Autodesk Inventor part; units mm, degrees
ref_plane "YZ Plane" through (0, 0, 0) normal (1, 0, 0) x (0, 1, 0)
ref_plane "XZ Plane" through (0, 0, 0) normal (0, 1, 0) x (-1, 0, 0)
ref_plane "XY Plane" through (0, 0, 0) normal (0, 0, 1) x (1, 0, 0)
sketch "Sketch1" plane through (0, 0, 0) normal (0, 1, 0) x (-1, 0, 0)
  line L0 (8.2338, 13.4805) -> (-21.7662, 13.4805)
  line L1 (-21.7662, 13.4805) -> (-21.7662, -11.5195)
  line L2 (-21.7662, -11.5195) -> (8.2338, -11.5195)
  line L3 (8.2338, -11.5195) -> (8.2338, 13.4805)
  point P0 (0, 0)
  dimension "d0" = 25
  dimension "d1" = 30
extrude "Extrusion1" add sketch "Sketch1" along normal blind 12.7
sketch "Sketch2" plane through (0, 0, 0) normal (0, -1, 0) x (1, 0, 0)
  line L0 (-8.2338, 13.4805) -> (21.7662, 13.4805)
  line L1 (21.7662, 13.4805) -> (21.7662, -11.5195)
  point P0 (0, 0)
  point P1 (19.2262, 10.3055)
  point P2 (19.2262, -8.7445)
  point P3 (-6.1738, -8.7445)
  point P4 (-6.1738, 10.3055)
  dimension "d4" = 3.175
  dimension "d5" = 2.54
  dimension "d6" = 19.05
  dimension "d7" = 2.54
  dimension "d8" = 25.4
  dimension "d9" = 3.175
  dimension "d10" = 19.05
  dimension "d11" = 0
hole "Hole1" at (19.2262, 0, 10.3055) at (19.2262, 0, -8.7445) at (-6.1738, 0, -8.7445) at (-6.1738, 0, 10.3055) direction (0, 1, 0) diameter 2.6416 depth 10 tip angle 118.188
sketch "Sketch3" plane through (0, 12.7, 0) normal (0, 1, 0) x (1, 0, 0)
  line L0 (-4.3838, -10.8805) -> (17.9162, -10.8805)
  line L1 (17.9162, -10.8805) -> (17.9162, 8.9195)
  line L2 (17.9162, 8.9195) -> (-4.3838, 8.9195)
  line L3 (-4.3838, 8.9195) -> (-4.3838, -10.8805)
  line L4 (-8.2338, 11.5195) -> (-8.2338, -13.4805)
  line L5 (21.7662, 11.5195) -> (-8.2338, 11.5195)
  point P0 (0, 0)
  dimension "d19" = 19.8
  dimension "d20" = 22.3
  dimension "d22" = 3.85
  dimension "d23" = 2.6
extrude "Extrusion2" cut sketch "Sketch3" against normal blind 1.57
sketch "Sketch4" plane through (0, 11.13, 0) normal (0, 1, 0) x (1, 0, 0)
  line L0 (-4.3838, -10.8805) -> (-4.3838, 8.9195)
  line L1 (17.9162, -10.8805) -> (-4.3838, -10.8805)
  line L2 (17.9162, 8.9195) -> (17.9162, -10.8805)
  point P0 (0, 0)
  point P1 (14.4162, -7.3805)
  point P2 (14.4162, 5.3195)
  point P3 (4.8762, 4.7295)
  point P4 (4.8762, -6.7005)
  dimension "d28" = 0
  dimension "d30" = 9.26
  dimension "d31" = 4.18
  dimension "d32" = 11.43
  dimension "d33" = 3.5
  dimension "d34" = 3.5
  dimension "d35" = 3.5
  dimension "d36" = 12.7
hole "Hole2" at (14.4162, 11.13, 7.3805) at (14.4162, 11.13, -5.3195) at (4.8762, 11.13, -4.7295) at (4.8762, 11.13, 6.7005) direction (0, -1, 0) diameter 2.4638 depth 6 tip angle 118.188
sketch "Sketch5" plane through (0, 11.13, 0) normal (0, 1, 0) x (1, 0, 0)
  line L0 (17.9162, -10.8805) -> (-4.3838, -10.8805)
  line L1 (-4.3838, -10.8805) -> (-4.3838, 8.9195)
  line L2 (0.4262, -0.8744) -> (4.9262, -3.4724)
  line L3 (4.9262, -3.4724) -> (4.9262, -8.6686)
  line L4 (4.9262, -8.6686) -> (0.4262, -11.2667)
  line L5 (0.4262, -11.2667) -> (-4.0738, -8.6686)
  line L6 (-4.0738, -8.6686) -> (-4.0738, -3.4724)
  line L7 (-4.0738, -3.4724) -> (0.4262, -0.8744)
  line L8 (0.4262, -1.1067) -> (-4.0738, 1.4914)
  line L9 (-4.0738, 1.4914) -> (-4.0738, 6.6876)
  line L10 (-4.0738, 6.6876) -> (0.4262, 9.2856)
  line L11 (0.4262, 9.2856) -> (4.9262, 6.6876)
  line L12 (4.9262, 6.6876) -> (4.9262, 1.4914)
  line L13 (4.9262, 1.4914) -> (0.4262, -1.1067)
  point P0 (0.4262, -6.0705)
  point P1 (0.4262, 4.0895)
  point P2 (0.4262, -6.0705)
  point P3 (0.4262, 4.0895)
  dimension "d49" = 4.81
  dimension "d50" = 4.81
  dimension "d51" = 10.16
  dimension "d52" = 0
  dimension "d53" = 9
  dimension "d54" = 9
extrude "Extrusion3" cut sketch "Sketch5" along normal mid plane 6.35
sketch "Sketch7" plane through (0, 7.955, 0) normal (0, 1, 0) x (1, 0, 0)
  line L0 (0.2251, -0.9905) -> (-4.0738, 1.4914)
  line L1 (-4.0738, -3.4724) -> (0.2251, -0.9905)
  line L2 (-4.0738, -8.6686) -> (-4.0738, -3.4724)
  line L3 (-0.2426, -10.8805) -> (-4.0738, -8.6686)
  line L4 (4.9262, -8.6686) -> (1.0951, -10.8805)
  line L5 (4.9262, -7.9314) -> (4.9262, -8.6686)
  line L6 (4.9262, -3.4724) -> (4.9262, -5.4696)
  line L7 (0.6274, -0.9905) -> (4.9262, -3.4724)
  line L8 (4.9262, 1.4914) -> (0.6274, -0.9905)
  line L9 (4.9262, 3.4986) -> (4.9262, 1.4914)
  line L10 (4.9262, 6.6876) -> (4.9262, 5.9604)
  line L11 (1.0604, 8.9195) -> (4.9262, 6.6876)
  line L12 (-4.0738, 6.6876) -> (-0.208, 8.9195)
  line L13 (-4.0738, 1.4914) -> (-4.0738, 6.6876)
  circle A0 centre (0.4262, -6.0705) radius 1.8986
  circle A1 centre (0.4262, 4.0895) radius 1.8986
  point P0 (0, 0)
  dimension "d57" = 3.7973
  dimension "d58" = 3.7973
extrude "Extrusion4" cut sketch "Sketch7" against normal blind 25.4
properties part number "CurrentMonitorBlock"
Could you check a few things on this model? Use its own coordinates, in mm. A direction names the side the tool comes from. Round coordinates to 2 decimals unless told otherwise and drop trailing zeros. Order: outer loops, then holes, each group sorted by start corner. A loop starts at its lowest first (then second) coordinate and runs counter-clockwise, first axis right, second up. Notation, with made-up numbers: M 78,56 L 87,56 A35 ccw 87,95 Z; hole C 26,24 d5. An arc over 180 degrees is marked long. One line per item, written item: value.
(1) Imagine slicing it at B-B (y = 5.5). Count the separate pieces of the cut face and the enclosed holes in it, and give its area (3 significant figures).
Ans:
separate pieces: 1
enclosed holes: 10
area: 686 mm^2
(2) I'm going to push flat-ended pins straight in: P1, Ø3, axis at x = 4.88, z = 6.7, coming from the +Y side; P2, Ø2.5, axis at x = 19.23, z = -8.74, coming from the -Y side; P3, Ø8, axis at x = -1.5, z = 1.5, coming from the +Y side. Where does each tip first touch, or does it pass through?
Ans:
P1: stops at y = 11.13
P2: stops at y = 10.04
P3: stops at y = 12.7
(3) If we mould it in two halves opening along Z, with no side actions, what happens to faces 1 (the conical face through (14.48, 4.52, -5.12)), 2 (the flat face through (21.766, 6, 1))? For each: released by +Z, released by -Z, zero draft, split by the parting line, or undercut.
Ans:
face 1: undercut
face 2: zero draft
(4) Which directions (+Z, -Z, +X, -X, +Y, -Y) give clear straight access to the entire face, cutting with the end or side of a thin tool? Please do faces 3 (the cylindrical face through (18.334, 5.07, 11.279)), 4 (the cylindrical face through (15.51, 8.09, -4.75)), 5 (the flat face through (7, 12.7, -10)).
Ans:
face 3: -Y
face 4: +Y
face 5: +Z, -Z, +X, -X, +Y
(5) Imagine slicing it at D-D (y = 8.75). Write out the boundary of the cut face in (x, z).
Ans:
outline: M -8.23,-11.52 L 21.77,-11.52 L 21.77,13.48 L -8.23,13.48 Z; hole C -6.17,-8.74 d2.64; hole C -6.17,10.31 d2.64; hole M -4.07,-6.69 L 0.43,-9.29 L 4.93,-6.69 L 4.93,-5.96 A1.23 ccw 4.93,-3.5 L 4.93,-1.49 L 0.63,0.99 L 4.93,3.47 L 4.93,5.47 A1.23 ccw 4.93,7.93 L 4.93,8.67 L 0.43,11.27 L -4.07,8.67 L -4.07,3.47 L 0.23,0.99 L -4.07,-1.49 Z; hole C 14.42,-5.32 d2.46; hole C 14.42,7.38 d2.46; hole C 19.23,-8.74 d2.64; hole C 19.23,10.31 d2.64
(6) I need wall thicknesses on line 1 along Z through (x, y) = (-4.25, 11.25); line 2 along X through (y, z) = (11.75, 1); line 3 along Z through (x, y) = (18.75, 4). Which ranges of each line are inside material? Lowest first, please. Write a range as from..to.
Ans:
line 1: z = -11.52..-8.92, 10.88..13.48
line 2: x = -8.23..-4.38, 17.92..21.77
line 3: z = -11.52..-9.98, -7.51..9.07, 11.54..13.48
(7) Imagine slicing it at C-C (z = -0.75). Write out the boundary of the cut face in (x, y) (3 decimals).
Ans:
outline: M -8.234,0 L 21.766,0 L 21.766,12.7 L 17.916,12.7 L 17.916,11.13 L 3.642,11.13 L 3.642,7.955 L -2.79,7.955 L -2.79,11.13 L -4.384,11.13 L -4.384,12.7 L -8.234,12.7 Z
(8) Imagine slicing it at A-A (x = 9). Write out the boundary of the cut face in (y, z), and give its area (3 significant figures).
Ans:
outline: M 0,-11.52 L 12.7,-11.52 L 12.7,-8.92 L 11.13,-8.92 L 11.13,10.88 L 12.7,10.88 L 12.7,13.48 L 0,13.48 Z
area: 286 mm^2
